```python
from build123d import *

# Parameters (mm, degrees)
SKETCH1_W                      = 14.8
SKETCH1_H                      = 20
SKETCH2_R                      = 13.85
BOSS_EXTRUDE1_DEPTH            = 12.9
BOSS_EXTRUDE2_DEPTH            = 6
BOSS_EXTRUDE3_DEPTH            = 6
BOSS_EXTRUDE4_START            = 4.9
SKETCH5_R                      = 13.85
BOSS_EXTRUDE4_DEPTH            = 4.9
SKETCH6_R                      = 5
BOSS_EXTRUDE5_DEPTH            = 2.6
SKETCH7_R                      = 1.15
BOSS_EXTRUDE6_DEPTH            = 7.8
BOSS_EXTRUDE7_START            = 2.6
SKETCH8_R                      = 5
BOSS_EXTRUDE7_DEPTH            = 2.6
BOSS_EXTRUDE8_START            = 11.2
SKETCH9_R                      = 1.15
BOSS_EXTRUDE8_DEPTH            = 11.2
F_2_6_2_6_DIAMETER_HOLE1_D     = 2.6
F_2_6_2_6_DIAMETER_HOLE1_DEPTH = 3.216319987
CHAMFER1_SIZE                  = 0.6
FILLET1_R                      = 1


with BuildPart() as part:
    # Sketch1 → Revolve1 (revolve)
    with BuildSketch(Plane.XZ, mode=Mode.PRIVATE) as revolve1_sk:
        with Locations((7.4, 22.9)):
            Rectangle(SKETCH1_W, SKETCH1_H)
    revolve(revolve1_sk.sketch.rotate(Axis((0, 0, 32.9), (0, 0, -1)), 270), axis=Axis((0, 0, 32.9), (0, 0, -1)))

    # Sketch2 → Boss-Extrude1 (add)
    with BuildSketch(Plane(origin=(0, 0, 12.9), x_dir=(-1, 0, 0), z_dir=(0, 0, -1))):
        with Locations(Location((0, 0, 0), (0, 0, 270))):
            Circle(SKETCH2_R)
    extrude(amount=BOSS_EXTRUDE1_DEPTH)

    # Sketch3 → Boss-Extrude2 (add)
    with BuildSketch(Plane(origin=(0, 0, 0), x_dir=(-1, 0, 0), z_dir=(0, 0, -1))):
        Polygon((-5.782608477, 10.080528964), (-2.666854949, 11.311211681), (-2.519907759, 10.939181409), (-5.635661287, 9.708498692), align=None)
    extrude(amount=BOSS_EXTRUDE2_DEPTH)

    # Sketch4 → Boss-Extrude3 (add)
    with BuildSketch(Plane(origin=(0, 0, 0), x_dir=(-1, 0, 0), z_dir=(0, 0, -1))):
        Polygon((2.519907759, -10.939181409), (5.635661287, -9.708498692), (5.782608477, -10.080528964), (2.666854949, -11.311211681), align=None)
    extrude(amount=BOSS_EXTRUDE3_DEPTH)

    # Sketch5 → Boss-Extrude4 (add)
    with BuildSketch(Plane.XY.offset(32.9).offset(BOSS_EXTRUDE4_START)):
        with Locations(Location((0, 0, 0), (0, 0, 270))):
            Circle(SKETCH5_R)
    extrude(amount=-BOSS_EXTRUDE4_DEPTH)

    # Sketch6 → Boss-Extrude5 (add)
    with BuildSketch(Plane.XY.offset(37.8)):
        Circle(SKETCH6_R)
    extrude(amount=BOSS_EXTRUDE5_DEPTH)

    # Sketch7 → Boss-Extrude6 (add)
    with BuildSketch(Plane.XY.offset(40.4)):
        Circle(SKETCH7_R)
    extrude(amount=BOSS_EXTRUDE6_DEPTH)

    # Sketch8 → Boss-Extrude7 (add)
    with BuildSketch(Plane(origin=(0, 0, 0), x_dir=(-1, 0, 0), z_dir=(0, 0, -1)).offset(BOSS_EXTRUDE7_START)):
        with Locations(Location((0, 0, 0), (0, 0, 180))):
            Circle(SKETCH8_R)
    extrude(amount=-BOSS_EXTRUDE7_DEPTH)

    # Sketch9 → Boss-Extrude8 (add)
    with BuildSketch(Plane(origin=(0, 0, -2.6), x_dir=(-1, 0, 0), z_dir=(0, 0, -1)).offset(BOSS_EXTRUDE8_START)):
        with Locations(Location((0, 0, 0), (0, 0, 180))):
            Circle(SKETCH9_R)
    extrude(amount=-BOSS_EXTRUDE8_DEPTH)

    # Ø2.6 (2.6) Diameter Hole1
    with Locations(Plane.XY.offset(37.8)):
        with Locations((-2.9389438, -7.440605442), (2.9389438, 7.440605442)):
            Hole(F_2_6_2_6_DIAMETER_HOLE1_D / 2, depth=F_2_6_2_6_DIAMETER_HOLE1_DEPTH)

    # Chamfer1
    chamfer1_edges = [part.edges().sort_by_distance(p)[0] for p in [
        (-5, 0, 40.4),
        (-5, 0, -2.6),
    ]]
    chamfer(chamfer1_edges, length=CHAMFER1_SIZE)

    # Fillet1
    fillet1_edges = [part.edges().sort_by_distance(p)[0] for p in [
        (0, 13.85, 37.8),
    ]]
    fillet(fillet1_edges, radius=FILLET1_R)


solid = part.part
```
Input: part model. Units: mm. Frame: model coordinates. A direction names the side the tool comes from. Give positions to 0.01 mm unless a question says otherwise; leave off trailing zeros. Loops run counter-clockwise (first coordinate to the right, second up) from the corner with the lowest first, then second, coordinate; pieces in that order, holes last.
1) Reachability of faces 1 (the cylindrical face through (-13.52, 3, 34.88)), 2 (the cylindrical face through (-5, 0, -1)), 3 (the flat face through (4.06, 10.33, -2.96)) from +Z, -Z, +X, -X, +Y, -Y: full face, straight path, thin tool, end or side. Return the list, or none.
A:
face 1: +Z
face 2: -Z
face 3: -Z, -X
2) Line query: L1, parallel to Z at x = 4, y = 6.25; L2, parallel to Z at x = 0.5, y = 2.5; L3, parallel to X at y = 0, z = 6. Output: solid intervals per line, ascending.
A:
L1: z = 0 to 37.8
L2: z = -2.6 to 40.4
L3: x = -13.85 to 13.85
3) Mould query, pull axis Y, two halves, no side actions, for faces 4 (the cylindrical face through (-14.448, -3.208, 23.04)), 5 (the flat face through (4.247, 10.687, -2.958)), 6 (the flat face through (3, 7, 34.584)). Classes: released by +Y, released by -Y, zero draft, split by the parting line, or undercut.
A:
face 4: split by the parting line
face 5: released by +Y
face 6: undercut
4) Contact query for flat-ended pins moving along their axis: pin 1 (2 mm diameter, centred on x = -2.94, y = -7.44, fed in from +Z); pin 2 (8 mm diameter, centred on x = 4, z = 4.5, fed in from -Y); pin 3 (1.3 mm diameter, centred on x = -3.5, y = -10, fed in from -Z). Output: stop coordinate, or through.
A:
pin 1: stops at z = 34.58
pin 2: stops at y = -13.85
pin 3: stops at z = -6
5) Section query C-C on z = 43. Return the cut outline in (x, y).
A:
outline: circle Ø2.3 at (0, 0)
